For this review, use the dimensioned drawing (mm, ordinates from the lowest corner) and the shaded views. Round coordinates to 2 decimals unless told otherwise and drop trailing zeros. Order: outer loops, then holes, each group sorted by start corner. A loop starts at its lowest first (then second) coordinate and runs counter-clockwise, first axis right, second up. Notation, with made-up numbers: (-38.75, -20.5) -> (-30.75, -20.5) arc R23 cw to (-30.75, 18.5) -> close; hole circle Ø2 at (84.5, -15.5). An arc over 180 degrees is marked (long way). Answer in a Markdown table with one row per item.
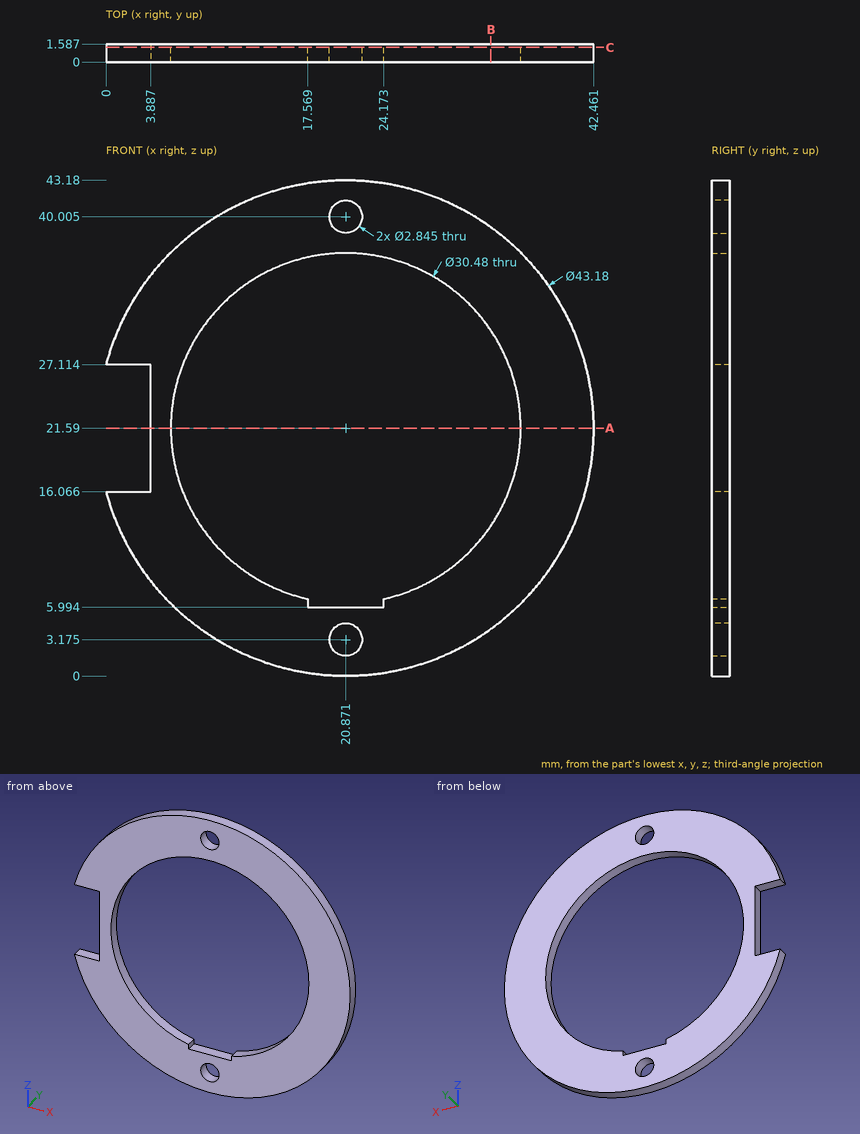
Q1. To check wall thickness, follow probe 1 along Z at (x, y) = (9.5, 0.2) (1 decimal); probe 2 along X at (y, z) = (0.4, 14.5) (1 decimal); probe 3 along Z at (x, y) = (18, 0.3) (1 decimal). State the ranges of each line that lie inside material, in increasing order.
Answer key:
| item | result |
|---|---|
| probe 1 | z = 3.2 to 11.4, 31.7 to 39.9 |
| probe 2 | x = 0.5 to 7.4, 34.4 to 41.3 |
| probe 3 | z = 0.2 to 6, 36.6 to 43 |
Q2. Take a section at B-B, the plane x = 33.5. Write out the cut boundary in (y, z).
Answer key:
| item | result |
|---|---|
| outline | (0, 4.08) -> (1.59, 4.08) -> (1.59, 13.06) -> (0, 13.06) -> close; (0, 30.12) -> (1.59, 30.12) -> (1.59, 39.1) -> (0, 39.1) -> close |
Q3. Take a section at C-C, the plane y = 1.3. Write out the cut boundary in (x, z) (1 decimal).
Answer key:
| item | result |
|---|---|
| outline | (0, 16.1) arc R21.6 ccw (long way) to (0, 27.1) -> (3.9, 27.1) -> (3.9, 16.1) -> close; hole (17.6, 6) -> (24.2, 6) -> (24.2, 6.7) arc R15.2 ccw (long way) to (17.6, 6.7) -> close; hole circle Ø2.8 at (20.9, 3.2); hole circle Ø2.8 at (20.9, 40) |
Q4. Clearance check with flat-ended pins moving along their axes: pin 1 Ø0.6 at (y, z) = (1, 6.5) entering from -X; pin 2 Ø0.5 at (y, z) = (1, 24) entering from -X; pin 3 Ø0.5 at (x, y) = (2.5, 1) entering from +Z (1 decimal). State where each tip first meets the part, or that it passes through.
Answer key:
| item | result |
|---|---|
| pin 1 | stops at x = 5.14 |
| pin 2 | stops at x = 3.89 |
| pin 3 | stops at z = 33.3 |
Q5. Take a section at A-A, the plane z = 21.59. Write out the cut boundary in (x, y).
Answer key:
| item | result |
|---|---|
| outline | (3.89, 0) -> (5.63, 0) -> (5.63, 1.59) -> (3.89, 1.59) -> close; (36.11, 0) -> (42.46, 0) -> (42.46, 1.59) -> (36.11, 1.59) -> close |
